The model under review builds one solid part; all positions refer to its coordinate system, in mm. Coordinates: 2 decimals unless noted, no trailing zeros. Write each loop counter-clockwise with the first axis right and the second up, starting at its lowest first coordinate (ties: lowest second). Pieces come first, ordered by that corner, then holes.
1) Add section C-C, the plane y = 3. Give the number of separate pieces and of enclosed holes in the cut face, then the cut area to 3 significant figures.
2) Mouldability with a two-part tool opening along X and no side actions: class faces 1 (the cylindrical face through (-315.248, 4.056, 121.986)), 2 (the flat face through (-333.47, 4, 143)), 3 (the flat face through (-269, 4, 207.409)), 4 (the flat face through (-203.47, 4, 143)) as released by +X, released by -X, zero draft, split by the parting line, or undercut.
3) For line 1 (Z direction, x = -218, y = 7); line 2 (Z direction, x = -315.5, y = 6.25); line 3 (X direction, y = 7, z = 124.5), list the stretches that pass through material, from the lowest coordinate up.
4) Add section B-B, the plane z = 156. State the section outline as (x, y) points.
5) Add section A-A, the plane x = -273. State the section outline as (y, z) points, then the cut area to 3 significant figures.
6) For P1, Ø10.5, axis at x = -318.47, z = 162.41, coming from the -Y side, flat-tipped, find the tip position at first contact; note if it passes through.
from build123d import *

# Parameters (mm, degrees)
SKETCH1_W             = 130
SKETCH1_H             = 130
SKETCH1_R             = 16.5
BOSS_EXTRUDE1_DEPTH   = 8
SKETCH2_R             = 3.25
CUT_EXTRUDE1_DEPTH    = 393.791233964
M6X1_0_TAPPED_HOLE2_D = 5


with BuildPart() as part:
    # Sketch1 → Boss-Extrude1 (new body)
    with BuildSketch(Plane(origin=(0, 0, 0), x_dir=(1, 0, 0), z_dir=(0, 1, 0))):
        with Locations((-268.470286077, -142.40906871)):
            Rectangle(SKETCH1_W, SKETCH1_H)
        with Locations(Location((-268.470286077, -142.40906871, 0), (0, 0, 270))):
            Circle(SKETCH1_R, mode=Mode.SUBTRACT)
    extrude(amount=BOSS_EXTRUDE1_DEPTH)

    # Sketch2 → Cut-Extrude1 (cut, through all)
    with BuildSketch(Plane(origin=(0, 8, 0), x_dir=(1, 0, 0), z_dir=(0, 1, 0))):
        with Locations(Location((-318.470286077, -162.40906871, 0), (0, 0, 270))):
            Circle(SKETCH2_R)
        with Locations(Location((-318.470286077, -122.40906871, 0), (0, 0, 270))):
            Circle(SKETCH2_R)
        with Locations(Location((-218.470286077, -122.40906871, 0), (0, 0, 270))):
            Circle(SKETCH2_R)
        with Locations(Location((-218.470286077, -162.40906871, 0), (0, 0, 270))):
            Circle(SKETCH2_R)
    extrude(amount=-CUT_EXTRUDE1_DEPTH, mode=Mode.SUBTRACT)

    # M6x1.0 Tapped Hole2 (through all)
    with Locations(Plane(origin=(0, 8, 0), x_dir=(1, 0, 0), z_dir=(0, 1, 0))):
        with Locations((-301.704286077, -109.17506871), (-235.236286077, -109.17506871), (-235.236286077, -175.64306871), (-301.704286077, -175.64306871)):
            Hole(M6X1_0_TAPPED_HOLE2_D / 2)


solid = part.part
Geometry results:
1. separate pieces: 1
1. enclosed holes: 9
1. area: 15,800 mm2
2. face 1: undercut
2. face 2: released by -X
2. face 3: zero draft
2. face 4: released by +X
3. line 1: z = 77.41 to 119.19, 125.62 to 159.19, 165.62 to 207.41
3. line 2: z = 77.41 to 121.09, 123.73 to 161.09, 163.73 to 207.41
3. line 3: x = -333.47 to -320.96, -315.98 to -220.96, -215.98 to -203.47
4. outline: (-333.47, 0) - (-277.83, 0) - (-277.83, 8) - (-333.47, 8) - close; (-259.11, 0) - (-203.47, 0) - (-203.47, 8) - (-259.11, 8) - close
5. outline: (0, 77.41) - (8, 77.41) - (8, 126.54) - (0, 126.54) - close; (0, 158.28) - (8, 158.28) - (8, 207.41) - (0, 207.41) - close
5. area: 786 mm2
6. P1: stops at y = 0
